Could you check a few things on this model? Use its own coordinates, in mm. A direction names the side the tool comes from. Give positions to 0.01 mm unless a question says otherwise; leave off trailing zeros. Write each loop counter-clockwise with the first axis right and the second up, starting at its lowest first coordinate (ties: lowest second). Pieces come first, ordered by that corner, then holes. Notation, with made-up numbers: (-3.75, 70.25) -> (18.25, 70.25) arc R28 ccw to (18.25, 108.25) -> close; hole circle Ø5 at (72, -18.75). An arc over 180 degrees is marked (long way). Write item = value, one per line. Start each with the question number.
```python
from build123d import *

# Parameters (mm, degrees)
SKETCH1_W           = 180
SKETCH1_H           = 145
BOSS_EXTRUDE1_DEPTH = 2.9
CUT_EXTRUDE1_DEPTH  = 124.929980231
SKETCH3_R           = 2.5
CUT_EXTRUDE2_DEPTH  = 124.929980231
SKETCH4_R           = 2.5
CUT_EXTRUDE3_DEPTH  = 124.929980231
FILLET1_R           = 10


with BuildPart() as part:
    # Sketch1 → Boss-Extrude1 (new, symmetric)
    with BuildSketch(Plane(origin=(0, 0, 0), x_dir=(1, 0, 0), z_dir=(0, 1, 0))):
        with Locations((0, -12.5)):
            Rectangle(SKETCH1_W, SKETCH1_H)
    extrude(amount=BOSS_EXTRUDE1_DEPTH, both=True)

    # Sketch2 → Cut-Extrude1 (cut, through all)
    with BuildSketch(Plane(origin=(0, 2.9, 0), x_dir=(1, 0, 0), z_dir=(0, 1, 0))):
        Polygon((-60, 23.8), (60, 23.8), (60, -23.8), (60, -36.74), (-60, -36.74), (-60, -23.8), align=None)
    extrude(amount=-CUT_EXTRUDE1_DEPTH, mode=Mode.SUBTRACT)

    # Sketch3 → Cut-Extrude2 (cut, through all)
    with BuildSketch(Plane(origin=(0, 2.9, 0), x_dir=(1, 0, 0), z_dir=(0, 1, 0))):
        with Locations(Location((-9.525, -44.36, 0), (0, 0, 270))):
            Circle(SKETCH3_R)
        with Locations(Location((9.525, -44.36, 0), (0, 0, 270))):
            Circle(SKETCH3_R)
        with Locations(Location((-9.525, -81.19, 0), (0, 0, 270))):
            Circle(SKETCH3_R)
        with Locations(Location((9.525, -81.19, 0), (0, 0, 270))):
            Circle(SKETCH3_R)
        with BuildLine():
            Line((-12.025, 30.889667183), (-12.025, 43.982098817))
            ThreePointArc((-12.025, 43.982098817), (-9.525, 46.482098817), (-7.025, 43.982098817))
            Line((-7.025, 43.982098817), (-7.025, 30.889667183))
            ThreePointArc((-7.025, 30.889667183), (-9.525, 28.389667183), (-12.025, 30.889667183))
        make_face()
        with BuildLine():
            Line((7.025, 30.889667183), (7.025, 43.982098817))
            ThreePointArc((7.025, 43.982098817), (9.525, 46.482098817), (12.025, 43.982098817))
            Line((12.025, 43.982098817), (12.025, 30.889667183))
            ThreePointArc((12.025, 30.889667183), (9.525, 28.389667183), (7.025, 30.889667183))
        make_face()
    extrude(amount=-CUT_EXTRUDE2_DEPTH, mode=Mode.SUBTRACT)

    # Sketch4 → Cut-Extrude3 (cut, through all)
    with BuildSketch(Plane(origin=(0, 2.9, 0), x_dir=(1, 0, 0), z_dir=(0, 1, 0))):
        with Locations(Location((-80, 50, 0), (0, 0, 270))):
            Circle(SKETCH4_R)
        with Locations(Location((-80, 3.99826174, 0), (0, 0, 270))):
            Circle(SKETCH4_R)
        with Locations(Location((-80, -75, 0), (0, 0, 270))):
            Circle(SKETCH4_R)
        with Locations(Location((80, -75, 0), (0, 0, 270))):
            Circle(SKETCH4_R)
        with Locations(Location((80, 3.99826174, 0), (0, 0, 270))):
            Circle(SKETCH4_R)
        with Locations(Location((80, 50, 0), (0, 0, 270))):
            Circle(SKETCH4_R)
    extrude(amount=-CUT_EXTRUDE3_DEPTH, mode=Mode.SUBTRACT)

    # Fillet1
    fillet1_edges = [part.edges().sort_by_distance(p)[0] for p in [
        (-60, 0, -23.8),
        (60, 0, -23.8),
        (60, 0, 36.74),
        (-60, 0, 36.74),
        (90, 0, 85),
        (-90, 0, 85),
        (-90, 0, -60),
        (90, 0, -60),
    ]]
    fillet(fillet1_edges, radius=FILLET1_R)


solid = part.part
```
(1) Imagine slicing it at A-A (z = 44.36). Please give me the cut outline in (x, y) (3 decimals), then the cut area to 3 significant figures.
(2) Imagine slicing it at D-D (y = -0.6). State how many separate pieces and enclosed holes the cut face has, then the cut area to 3 significant figures.
(3) We'd pull the mould along X, two halves only. Please class faces 1 (the flat face through (90, 0, 13)), 2 (the flat face through (-1, 0, 85)), 3 (the cylindrical face through (56.99, -0.04, 33.89)), 4 (the flat face through (7.025, 0, -37)): released by +X, released by -X, zero draft, split by the parting line, or undercut.
(4) On a 3-axis mill with a long thin cutter (end or side, diameter ignored), from which of +Z, -Z, +X, -X, +Y, -Y can I reach the whole of each face in a straight line? I mean faces 5 (the flat face through (-1, -2.9, 44)), 6 (the flat face through (-7.025, 0, -38)). Say none if no direction works.
(5) Imagine slicing it at B-B (x = 36). Please give me the cut outline in (y, z), then the cut area to 3 significant figures.
(6) If I drill on line 1 along X through (y, z) = (0.95, -50); line 2 along X through (y, z) = (0.65, 44.36) (3 decimals); line 3 along X through (y, z) = (0.35, 7), over which ranges is the centre line in solid material (lowest first)? Write a range as from..to.
(7) Imagine slicing it at C-C (z = 10.5). Please give me the cut outline in (x, y).
Answers below:
q1.outline = (-90, -2.9) -> (-12.025, -2.9) -> (-12.025, 2.9) -> (-90, 2.9) -> close; (-7.025, -2.9) -> (7.025, -2.9) -> (7.025, 2.9) -> (-7.025, 2.9) -> close; (12.025, -2.9) -> (90, -2.9) -> (90, 2.9) -> (12.025, 2.9) -> close
q1.area = 986 mm^2
q2.separate_pieces = 1
q2.enclosed_holes = 13
q2.area = 18,500 mm^2
q3.face_1 = released by +X
q3.face_2 = zero draft
q3.face_3 = undercut
q3.face_4 = undercut
q4.face_5 = +Z, -Z, +X, -X, -Y
q4.face_6 = +Y, -Y
q5.outline = (-2.9, -60) -> (2.9, -60) -> (2.9, -23.8) -> (-2.9, -23.8) -> close; (-2.9, 36.74) -> (2.9, 36.74) -> (2.9, 85) -> (-2.9, 85) -> close
q5.area = 490 mm^2
q6.line_1 = -90..-82.5, -77.5..77.5, 82.5..90
q6.line_2 = -90..-12.025, -7.025..7.025, 12.025..90
q6.line_3 = -90..-60, 60..90
q7.outline = (-90, -2.9) -> (-60, -2.9) -> (-60, 2.9) -> (-90, 2.9) -> close; (60, -2.9) -> (90, -2.9) -> (90, 2.9) -> (60, 2.9) -> close
